CAD build for the part. Positions are in the model's coordinates, mm. A direction names the side the tool comes from. Round coordinates to 2 decimals unless told otherwise and drop trailing zeros. Loops run counter-clockwise (first coordinate to the right, second up) from the corner with the lowest first, then second, coordinate; pieces in that order, holes last. Notation, with made-up numbers: (82, 45.25) - (119, 45.25) arc R36 cw to (119, 82.25) - close; hole circle Ø6 at (37, -13). An arc over 180 degrees is marked (long way). One line per question, with ' | ' between items.
```python
from build123d import *

# Parameters (mm, degrees)
F0_W     = 7
F0_H     = 7
F1_DEPTH = 11.5
F2_W     = 5.5
F2_H     = 5.5
F3_DEPTH = 14


with BuildPart() as f1:
    # F0 (on Right) → F1 (new body)
    with BuildSketch(Plane.YZ):
        with Locations((3.5, 3.5)):
            Rectangle(F0_W, F0_H)
    extrude(amount=F1_DEPTH)

    # F2 (on face) → F3 (join)
    with BuildSketch(Plane.YZ.offset(11.5)):
        with Locations((3.5, 3.5)):
            Rectangle(F2_W, F2_H)
    extrude(amount=F3_DEPTH)

    # F4: F1 across face


with BuildPart() as f1_1:
    add(f1.part)
    add(f1.part.mirror(Plane(origin=(0, 3.5, 3.5), x_dir=(0, 1, 0), z_dir=(-1, 0, 0))))


solid = f1_1.part
```
(1) Tool access for faces 1 (the face through (-18, 3, 0.75)), 2 (the face through (-18, 0.75, 3)), 3 (the face through (18, 0.75, 3)), 4 (the face through (-18, 6.25, 3)), 5 (the face through (18, 6.25, 3)): list every direction of +Z, -Z, +X, -X, +Y, -Y with a clear straight run to the whole face (end or side of a thin tool).
Results found:
face 1: -Z, -X, +Y, -Y | face 2: +Z, -Z, -X, -Y | face 3: +Z, -Z, +X, -Y | face 4: +Z, -Z, -X, +Y | face 5: +Z, -Z, +X, +Y
(2) Probe L1, parallel to X at y = 0.5, z = 6.75; L2, parallel to Y at x = -12, z = 3.75. List the from-to ranges inside material, lowest first.
Results found:
L1: x = -11.5 to 11.5 | L2: y = 0.75 to 6.25
(3) Drop flat-ended pins along their axis: P1, Ø1.6, axis at x = -17.5, y = 3, coming from the -Z side; P2, Ø3, axis at x = 16.5, y = 4.5, coming from the +Z side; P3, Ø1.6, axis at x = 21, z = 3.5, coming from the -Y side. Give the stop position or say it passes through.
Results found:
P1: stops at z = 0.75 | P2: stops at z = 6.25 | P3: stops at y = 0.75
(4) Cut at C-C, the plane x = 20.5. Write the cut outline in (y, z).
Results found:
outline: (0.75, 0.75) - (6.25, 0.75) - (6.25, 6.25) - (0.75, 6.25) - close
(5) Cut at A-A, the plane z = 1.75. Write the cut outline in (x, y), then the cut area to 3 significant figures.
Results found:
outline: (-25.5, 0.75) - (-11.5, 0.75) - (-11.5, 0) - (11.5, 0) - (11.5, 0.75) - (25.5, 0.75) - (25.5, 6.25) - (11.5, 6.25) - (11.5, 7) - (-11.5, 7) - (-11.5, 6.25) - (-25.5, 6.25) - close | area: 315 mm²
